Read the model definition and answer for the solid it produces. Units are mm, in the model's axes. A direction names the side the tool comes from. Coordinates: 2 decimals unless noted, no trailing zeros. Order: outer loops, then holes, each group sorted by start corner. A loop starts at its lowest first (then second) coordinate and runs counter-clockwise, first axis right, second up. Notation, with made-up numbers: (37.5, -9) -> (94.5, -9) arc R4 cw to (94.5, -3) -> close; hole circle Ø11 at (82, -22). An arc over 180 degrees is marked (long way). Answer as a JSON object with one key per item and string values. Group by question number.
1) Given pin 1 (5 mm diameter, centred on y = -5.5, z = 4, fed in from -X); pin 2 (10 mm diameter, centred on x = -13, z = -7, fed in from -Y); pin 3 (1 mm diameter, centred on y = 9, z = 6, fed in from -X), each flat-ended and moving along its own axis, determine where each tip first touches the part or whether it passes through.
2) Determine the mould class of faces 3 (the cylindrical face through (1.19, 5.37, -0.28)), 4 (the conical face through (-22.758, -7.167, 14.464)), 5 (the flat face through (0, 6, 20)), 6 (the conical face through (-21.523, -6.778, 11.607)) for opening direction Z: released by +Z, released by -Z, zero draft, split by the parting line, or undercut.
3) Consider L1, parallel to Y at x = -14.5, z = -0.5; L2, parallel to Y at x = 0, z = 9; L3, parallel to Y at x = -5, z = 18. Determine where each line is inside the solid, lowest interval first.
4) Section A-A on y = 0 is taken. Determine the outline of the cut face in (x, z), and give its area (3 significant figures).
5) Section D-D on z = 16 is taken. Determine the outline of the cut face in (x, y).
6) A tool of negligible diameter and unlimited length cuts with its end or side. For faces 1 (the flat face through (0, 6, -20)), 2 (the conical face through (-9.65, 18.55, 5.89)), from which of +Z, -Z, +X, -X, +Y, -Y can it reach the whole face along a straight path? Write none if from no direction.
7) Section C-C on z = -1.5 is taken. Determine the outline of the cut face in (x, y).
from build123d import *


with BuildPart() as part:
    # Revolve profile 1 → Revolve 1 (revolve)
    with BuildSketch(Plane(origin=(0, 0, 0), x_dir=(1, 0, 0), z_dir=(0, 1, 0)), mode=Mode.PRIVATE) as revolve_1_sk:
        with BuildLine():
            Line((5.5, -20), (5.5, 20))
            Line((5.5, 20), (27.469967387, 20))
            Line((27.469967387, 20), (25.394644355, 17.142857143))
            Line((25.394644355, 17.142857143), (23.757463511, 14.285714286))
            Line((23.757463511, 14.285714286), (22.485423007, 11.428571429))
            Line((22.485423007, 11.428571429), (21.532753452, 8.571428571))
            Line((21.532753452, 8.571428571), (20.87011984, 5.714285714))
            ThreePointArc((20.87011984, 5.714285714), (20.35, 0), (20.87011984, -5.714285714))
            Line((20.87011984, -5.714285714), (21.532753452, -8.571428571))
            Line((21.532753452, -8.571428571), (22.485423007, -11.428571429))
            Line((22.485423007, -11.428571429), (23.757463511, -14.285714286))
            Line((23.757463511, -14.285714286), (25.394644355, -17.142857143))
            Line((25.394644355, -17.142857143), (27.469967387, -20))
            Line((27.469967387, -20), (5.5, -20))
        make_face()
    revolve(revolve_1_sk.sketch.rotate(Axis((0, 0, -25), (0, 0, 1)), 180), axis=Axis((0, 0, -25), (0, 0, 1)))


solid = part.part
Worked answers:
{
 "1": {"pin 1": "stops at x = -20.55", "pin 2": "stops at y = -20.09", "pin 3": "stops at x = -19.17"},
 "2": {"face 3": "zero draft", "face 4": "undercut", "face 5": "released by +Z", "face 6": "undercut"},
 "3": {"L1": "y = -14.28 to 14.28", "L2": "y = -21.68 to -5.5, 5.5 to 21.68", "L3": "y = -25.53 to -2.29, 2.29 to 25.53"},
 "4": {"outline": "(-27.47, -20) -> (-5.5, -20) -> (-5.5, 20) -> (-27.47, 20) -> (-25.39, 17.14) -> (-23.76, 14.29) -> (-22.49, 11.43) -> (-21.53, 8.57) -> (-20.87, 5.71) arc R31.65 cw to (-20.87, -5.71) -> (-21.53, -8.57) -> (-22.49, -11.43) -> (-23.76, -14.29) -> (-25.39, -17.14) -> close; (5.5, -20) -> (27.47, -20) -> (25.39, -17.14) -> (23.76, -14.29) -> (22.49, -11.43) -> (21.53, -8.57) -> (20.87, -5.71) arc R31.65 cw to (20.87, 5.71) -> (21.53, 8.57) -> (22.49, 11.43) -> (23.76, 14.29) -> (25.39, 17.14) -> (27.47, 20) -> (5.5, 20) -> close", "area": "1,370 mm²"},
 "5": {"outline": "circle Ø49.48 at (0, 0); hole circle Ø11 at (0, 0)"},
 "6": {"face 1": "-Z, +X, -X, +Y, -Y", "face 2": "none"},
 "7": {"outline": "circle Ø40.77 at (0, 0); hole circle Ø11 at (0, 0)"}
}
